Verification items for this drawing (mm, ordinates from the low corner). A direction names the side the tool comes from. Round coordinates to 2 decimals unless told otherwise and drop trailing zeros. Loops run counter-clockwise (first coordinate to the right, second up) from the corner with the lowest first, then second, coordinate; pieces in that order, holes last. Notation, with made-up numbers: (24.25, -27) - (63.25, -27) arc R11 cw to (63.25, -11) - close; hole circle Ø6 at (-27, 61). An arc over 180 degrees is marked (long way). Write item = value, one per line.
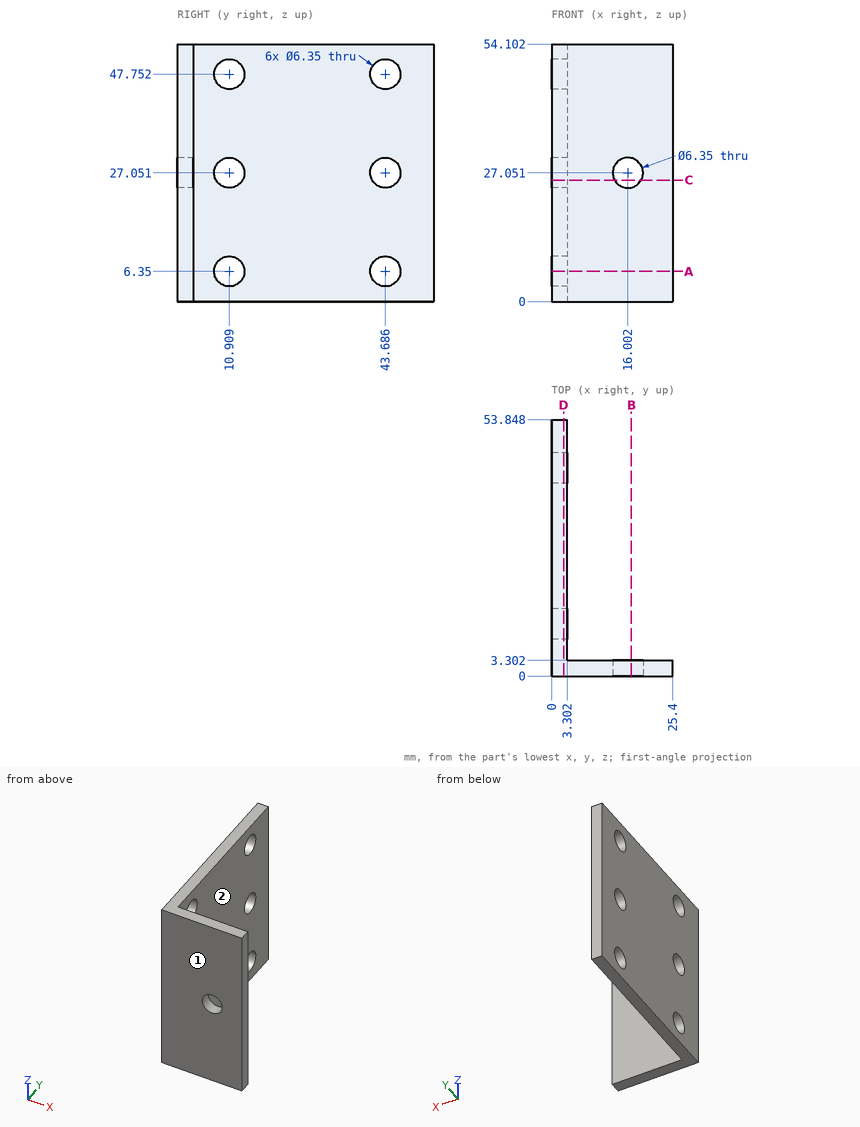
(1) Scan lines: L1, parallel to Y at x = 1.05, z = 6.35 (1 decimal); L2, parallel to X at y = 36.5, z = 45. Record each from-to range of solid material in increasing order. Write a range as [from, to].
Answers follow:
L1 = [0, 7.7], [14.1, 40.5], [46.9, 53.8]
L2 = [0, 3.3]
(2) Section check D-D (x = 2.5). State how many separate pieces and enclosed holes the cut face has, then the cut area to 3 significant figures.
Answers follow:
separate_pieces = 1
enclosed_holes = 6
area = 2,720 mm²
(3) Section check A-A (z = 6.35). Enter the section's corners in (x, y) (1 decimal).
Answers follow:
outline = (0, 0) - (25.4, 0) - (25.4, 3.3) - (3.3, 3.3) - (3.3, 7.7) - (0, 7.7) - close; (0, 14.1) - (3.3, 14.1) - (3.3, 40.5) - (0, 40.5) - close; (0, 46.9) - (3.3, 46.9) - (3.3, 53.8) - (0, 53.8) - close
(4) Set-up check for the marked faces 1 and 2: record each of +Z, -Z, +X, -X, +Y, -Y from which the full face is reachable in a straight line by a thin tool's end or side.
Answers follow:
face_1 = +Z, -Z, +X, -X, -Y
face_2 = +Z, -Z, +X, +Y
(5) Section check C-C (z = 25.5). Enter the section's corners in (x, y) (1 decimal).
Answers follow:
outline = (0, 0) - (13.2, 0) - (13.2, 3.3) - (3.3, 3.3) - (3.3, 8.1) - (0, 8.1) - close; (0, 13.7) - (3.3, 13.7) - (3.3, 40.9) - (0, 40.9) - close; (0, 46.5) - (3.3, 46.5) - (3.3, 53.8) - (0, 53.8) - close; (18.8, 0) - (25.4, 0) - (25.4, 3.3) - (18.8, 3.3) - close
(6) Section check B-B (x = 16.75). Enter the section's corners in (y, z) (1 decimal), then the cut area to 3 significant figures.
Answers follow:
outline = (0, 0) - (3.3, 0) - (3.3, 24) - (0, 24) - close; (0, 30.1) - (3.3, 30.1) - (3.3, 54.1) - (0, 54.1) - close
area = 158 mm²
(7) Gauge pin test, flat ends, axial feed: pin 1 (7.5 mm diameter, centred on y = 43.69, z = 47.75, fed in from +X); pin 2 (12 mm diameter, centred on x = 21, z = 42, fed in from +Y). Record the tip position at first contact, or that the pin passes through.
Answers follow:
pin_1 = 3.3
pin_2 = 3.3
